```python
from build123d import *

# Parameters (mm, degrees)
F0_W     = 30
F0_H     = 30
F1_DEPTH = 10
F2_DEPTH = 30


with BuildPart() as f1:
    # F0 (on Top) → F1 (new body)
    with BuildSketch(Plane.XY):
        with Locations((-29.82143, -25.982142)):
            Rectangle(F0_W, F0_H)
    extrude(amount=F1_DEPTH)

    # F0 (on Top) → F2 (join)
    with BuildSketch(Plane.XY):
        Polygon((-53.82143, -26.982142), (-53.82143, -40.982142), (-44.82143, -40.982142), (-44.82143, -10.982142), (-64.82143, -10.982142), (-64.82143, -26.982142), align=None)
        Polygon((-14.82143, -10.982142), (-14.82143, -40.982142), (-5.82143, -40.982142), (-5.82143, -26.982142), (5.17857, -26.982142), (5.17857, -10.982142), align=None)
    extrude(amount=F2_DEPTH)


solid = f1.part
```
Could you check a few things on this model? Use its own coordinates, in mm. A direction names the side the tool comes from. Give positions to 0.01 mm unless a question says otherwise; leave off trailing zeros. Loops run counter-clockwise (first coordinate to the right, second up) from the corner with the lowest first, then second, coordinate; pieces in that order, holes last. Notation, with made-up numbers: (58, 37) - (94, 37) arc R19 cw to (94, 54) - close; hole circle Ø6 at (18.5, 37). An arc over 180 degrees is marked (long way). Answer in a Markdown table with one row per item. Add a question column.
Q1. If we section it at C-C (z = 7.25): List the corners of the cut face in (x, y) for me.
Q2. If we section it at B-B (y = -21.5): List the corners of the cut face in (x, z) for me.
Q3. We'd pull the mould along X, two halves only. Please class faces 1 (the face through (-44.821, -26, 20)), 2 (the face through (0, -26.982, 15)), 3 (the face through (-53.821, -34, 15)): +X half, -X half, draft (parallel to the pull), parting line (faces both ways), or undercut.
Q4. Please list where these lines run through material, in increasing order: L1, parallel to X at y = -29, z = 13.5; L2, parallel to Z at x = -32.5, y = -28; L3, parallel to X at y = -22, z = 28.5. Write a range as from..to.
Q5. Which directions (+Z, -Z, +X, -X, +Y, -Y) give clear straight access to the entire face, cutting with the end or side of a thin tool? Please do faces 4 (the face through (-5.821, -34, 15)), 5 (the face through (-53, -22, 30)), 6 (the face through (-59, -26.982, 15)), 7 (the face through (-30, -26, 10)).
Q6. If we section it at D-D (x = -4.5): List the corners of the cut face in (y, z) for me, plus the area to 3 significant figures.
Q7. If we section it at A-A (z = 19): List the corners of the cut face in (x, y) for me.
Q8. For pin 1 (11 mm diameter, centred on y = -36, z = 16, fed in from +X); pin 2 (3.5 mm diameter, centred on x = -60.5, z = 16.5, fed in from -Y); pin 3 (4 mm diameter, centred on x = -32.5, y = -24, fed in from +Z), each with a flat end and sliding along its axis, tell me the tip position at first contact or that it passes through.
The answers:
| question | item | result |
|---|---|---|
| 1 | outline | (-64.82, -26.98) - (-53.82, -26.98) - (-53.82, -40.98) - (-5.82, -40.98) - (-5.82, -26.98) - (5.18, -26.98) - (5.18, -10.98) - (-64.82, -10.98) - close |
| 2 | outline | (-64.82, 0) - (5.18, 0) - (5.18, 30) - (-14.82, 30) - (-14.82, 10) - (-44.82, 10) - (-44.82, 30) - (-64.82, 30) - close |
| 3 | face 1 | undercut |
| 3 | face 2 | draft |
| 3 | face 3 | -X half |
| 4 | L1 | x = -53.82..-44.82, -14.82..-5.82 |
| 4 | L2 | z = 0..10 |
| 4 | L3 | x = -64.82..-44.82, -14.82..5.18 |
| 5 | face 4 | +Z, -Z, +X, -Y |
| 5 | face 5 | +Z, +X, -X, +Y, -Y |
| 5 | face 6 | +Z, -Z, -X, -Y |
| 5 | face 7 | +Z, +Y, -Y |
| 6 | outline | (-26.98, 0) - (-10.98, 0) - (-10.98, 30) - (-26.98, 30) - close |
| 6 | area | 480 mm^2 |
| 7 | outline | (-64.82, -26.98) - (-53.82, -26.98) - (-53.82, -40.98) - (-44.82, -40.98) - (-44.82, -10.98) - (-64.82, -10.98) - close; (-14.82, -40.98) - (-5.82, -40.98) - (-5.82, -26.98) - (5.18, -26.98) - (5.18, -10.98) - (-14.82, -10.98) - close |
| 8 | pin 1 | stops at x = -5.82 |
| 8 | pin 2 | stops at y = -26.98 |
| 8 | pin 3 | stops at z = 10 |
